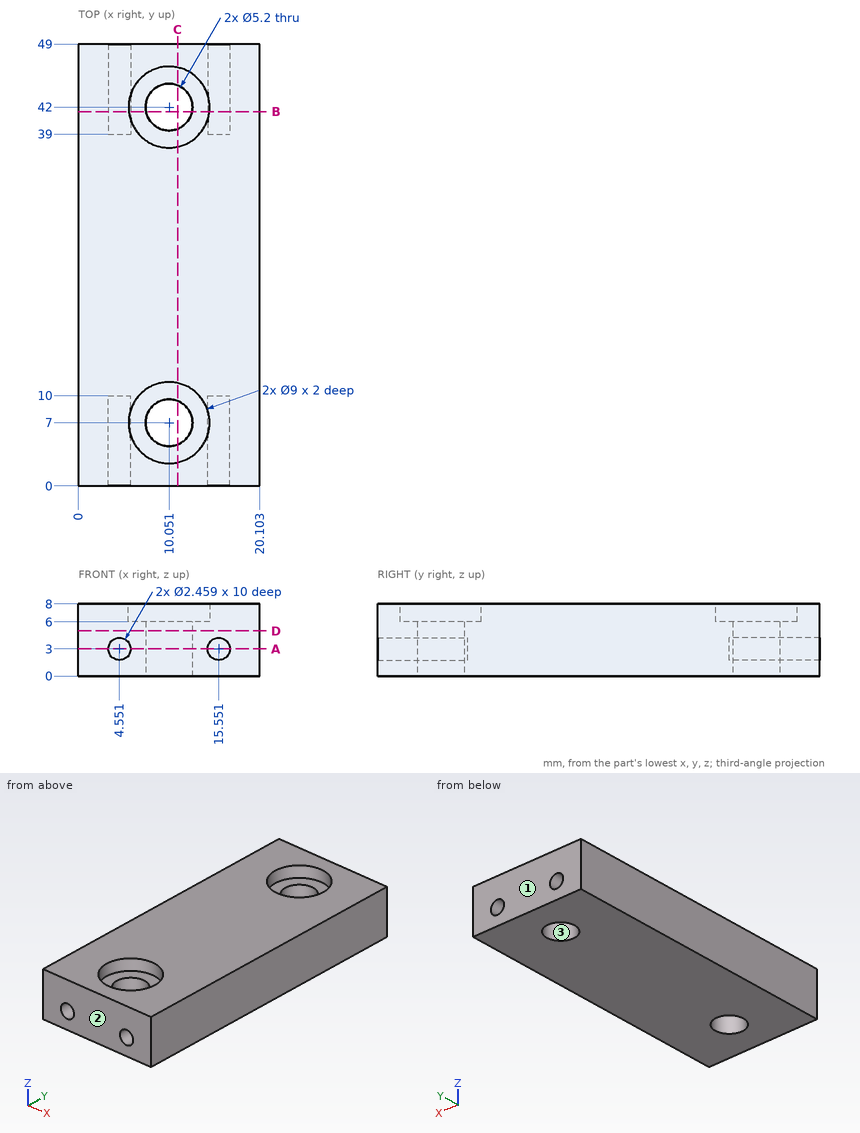
Can you work these out from the drawing? Everything is in mm from the part's minimum corner. Coordinates: 2 decimals unless noted, no trailing zeros. Loops run counter-clockwise (first coordinate to the right, second up) from the corner with the lowest first, then second, coordinate; pieces in that order, holes last. Notation, with made-up numbers: M 61.5,37 L 85.5,37 A15 cw 85.5,56 Z; hole C 85,84.5 d6. An arc over 180 degrees is marked long. Put each result on its own line as item: value. Start each with the question number.
(1) Thinking about a two-plate mould opening in Y: for the marked faces 1, 2 and 3, which applies, pulls with the +Y half, pulls with the -Y half, needs draft (parallel to the pull), parting line crosses it, or undercut?
(2) Suppose I cut it at A-A on z = 3. Please give me the cut outline in (x, y).
(3) Suppose I cut it at D-D on z = 5. Please give me the cut outline in (x, y).
(4) Suppose I cut it at C-C on x = 11. Please give me the cut outline in (y, z), then the cut area to 3 significant figures.
(5) Will these pins go through, and if not, where does the flat tip stop? P1, Ø0.7, axis at x = 4.5, z = 3, coming from the +Y side; P2, Ø8.5, axis at x = 10.05, y = 7, coming from the +Z side; P3, Ø0.7, axis at x = 16, z = 3, coming from the -Y side.
(6) I need wall thicknesses on line 1 (Y direction, x = 10, z = 1.25); line 2 (Y direction, x = 12, z = 5); line 3 (X direction, y = 44, z = 3.5) (1 decimal). Which ranges of each line are inside material? Lowest first, please. Write a range as from..to.
(7) Suppose I cut it at B-B on y = 41.5. Please give me the cut outline in (x, z).
Solutions:
1. face 1: pulls with the +Y half
1. face 2: pulls with the -Y half
1. face 3: undercut
2. outline: M 0,0 L 3.32,0 L 3.32,10 L 5.78,10 L 5.78,0 L 14.32,0 L 14.32,10 L 16.78,10 L 16.78,0 L 20.1,0 L 20.1,49 L 16.78,49 L 16.78,39 L 14.32,39 L 14.32,49 L 5.78,49 L 5.78,39 L 3.32,39 L 3.32,49 L 0,49 Z; hole C 10.05,7 d5.2; hole C 10.05,42 d5.2
3. outline: M 0,0 L 20.1,0 L 20.1,49 L 0,49 Z; hole C 10.05,7 d5.2; hole C 10.05,42 d5.2
4. outline: M 0,0 L 4.58,0 L 4.58,6 L 2.6,6 L 2.6,8 L 0,8 Z; M 9.42,0 L 39.58,0 L 39.58,6 L 37.6,6 L 37.6,8 L 11.4,8 L 11.4,6 L 9.42,6 Z; M 44.42,0 L 49,0 L 49,8 L 46.4,8 L 46.4,6 L 44.42,6 Z
4. area: 299 mm2
5. P1: stops at y = 39
5. P2: stops at z = 6
5. P3: stops at y = 10
6. line 1: y = 0..4.4, 9.6..39.4, 44.6..49
6. line 2: y = 0..5.28, 8.72..40.28, 43.72..49
6. line 3: x = 0..3.4, 5.7..8.4, 11.7..14.4, 16.7..20.1
7. outline: M 0,0 L 7.5,0 L 7.5,6 L 5.58,6 L 5.58,8 L 0,8 Z; M 12.6,0 L 20.1,0 L 20.1,8 L 14.52,8 L 14.52,6 L 12.6,6 Z; hole C 4.55,3 d2.46; hole C 15.55,3 d2.46
